For this review, use the dimensioned drawing (mm, ordinates from the lowest corner) and the shaded views. Give positions to 0.01 mm unless a question says otherwise; leave off trailing zeros. Loops run counter-clockwise (first coordinate to the right, second up) from the corner with the lowest first, then second, coordinate; pieces in that order, holes last. Notation, with made-up numbers: M 69.5,17 L 119.5,17 A11 cw 119.5,26 Z; hole C -33,16 d6. An arc over 180 degrees is marked long. Use CSV: the item, a comma, the result in double quotes.
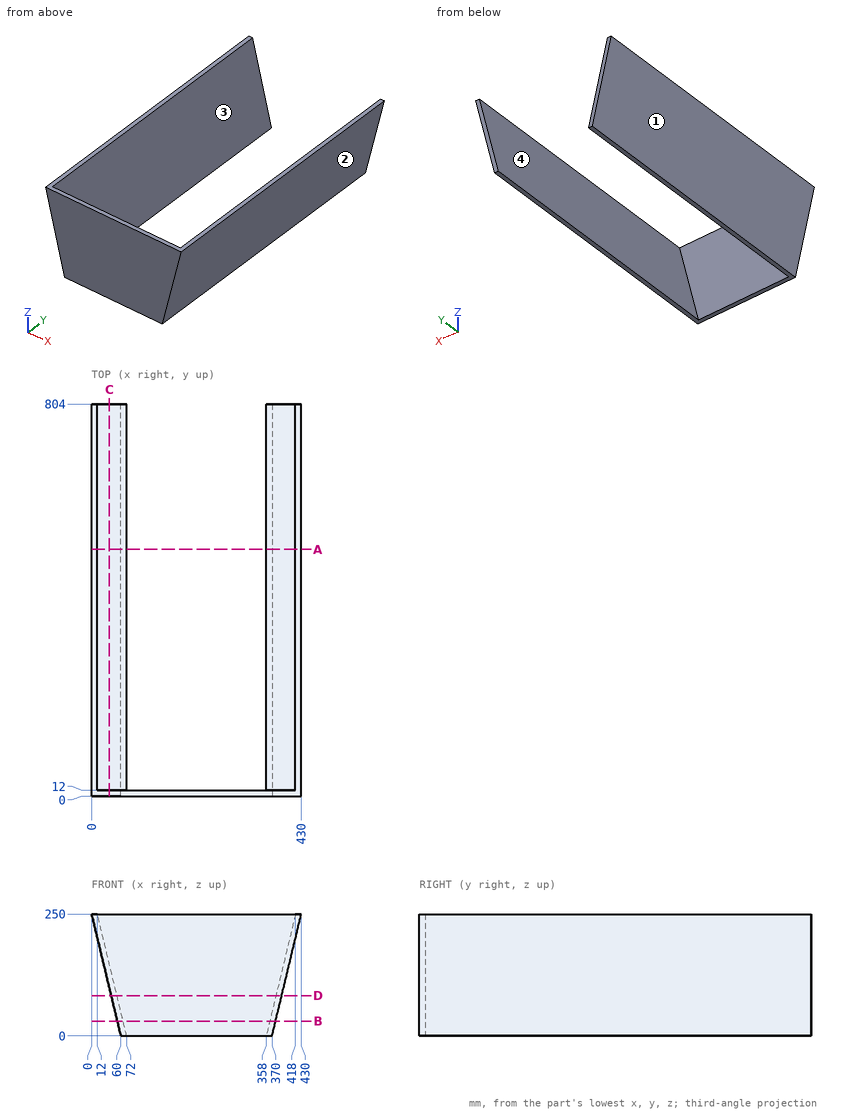
(1) The part is to be moulded in two halves that separate along X. For the marked faces 1, 2, 3 and 4, say which applies: released by +X, released by -X, zero draft, split by the parting line, or undercut.
A:
face 1,"released by -X"
face 2,"released by +X"
face 3,"undercut"
face 4,"undercut"
(2) Wall thickness on line 1 along Y through (x, z) = (342, 64.5); line 2 along X through (y, z) = (151, 11); line 3 along X through (y, z) = (273, 136.5): over which ranges is each line inside the solid? List them lowest first. Write a range as [from, to].
A:
line 1,"[0, 12]"
line 2,"[57.36, 69.36], [360.64, 372.64]"
line 3,"[27.24, 39.24], [390.76, 402.76]"
(3) Clearance check with flat-ended pins moving along their axes: P1, Ø1, axis at y = 436.5, z = 53, coming from the +X side; P2, Ø5, axis at x = 254.5, z = 212, coming from the +Y side; P3, Ø4, axis at y = 705.5, z = 191.5, coming from the -X side. State where each tip first meets the part, or that it passes through.
A:
P1,"x = 382.84"
P2,"y = 12"
P3,"x = 13.56"
(4) We need section D-D on z = 83. State the section outline as (x, y) points.
A:
outline,"M 40.08,0 L 389.92,0 L 389.92,804 L 377.92,804 L 377.92,12 L 52.08,12 L 52.08,804 L 40.08,804 Z"
(5) We need section B-B on z = 30.5. State the section outline as (x, y) points, then the cut area to 3 significant figures.
A:
outline,"M 52.68,0 L 377.32,0 L 377.32,804 L 365.32,804 L 365.32,12 L 64.68,12 L 64.68,804 L 52.68,804 Z"
area,"22,900 mm²"
(6) We need section C-C on x = 36.5. State the section outline as (y, z) points, then the cut area to 3 significant figures.
A:
outline,"M 0,97.92 L 804,97.92 L 804,147.92 L 12,147.92 L 12,250 L 0,250 Z"
area,"41,400 mm²"
(7) We need section A-A on y = 506. State the section outline as (x, z) points, then the cut area to 3 significant figures.
A:
outline,"M 0,250 L 60,0 L 72,0 L 12,250 Z; M 358,0 L 370,0 L 430,250 L 418,250 Z"
area,"6,000 mm²"
